```python
from build123d import *

# Parameters (mm, degrees)
F3_D     = 10
F3_DEPTH = 18


with BuildPart() as f1:
    # F0 (on Top) → F1 (revolve)
    with BuildSketch(Plane.XY):
        Polygon((0, 42.5), (0, 9), (85, 9), (85, 14), (48, 21), (18, 21), (18, 42.5), align=None)
    revolve(axis=Axis((69.263607, 0, 0), (1, 0, 0)))

    # F3
    with Locations(Plane.YZ.offset(18)):
        with Locations((0, 32.5), (-32.5, 0), (0, -32.5), (32.5, 0)):
            Hole(F3_D / 2, depth=F3_DEPTH)


solid = f1.part
```
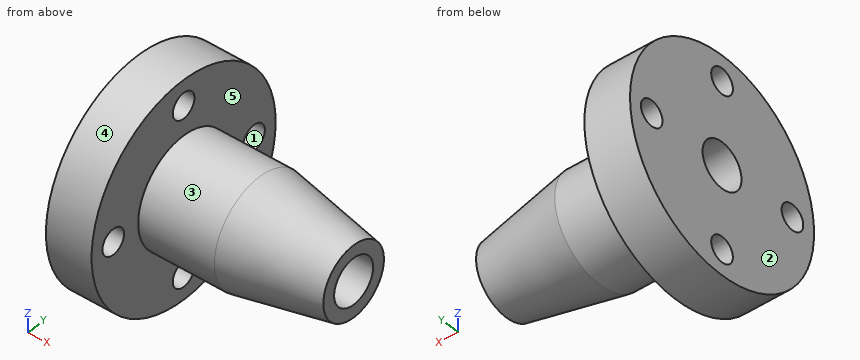
Geometry check sheet. Reference: the model listing, model coordinates, mm. Face numbers are marked on the shaded views. A direction names the side the tool comes from. Coordinates: 2 decimals unless noted, no trailing zeros. Order: outer loops, then holes, each group sorted by start corner. A loop starts at its lowest first (then second) coordinate and runs counter-clockwise, first axis right, second up. Notation, with made-up numbers: M 20.25,45 L 24.25,45 A28 cw 24.25,72 Z; hole C 6.25,2.25 d10. An arc over 180 degrees is marked long. Answer as a JSON object with one key per item and string values.
Q1. Cross-section at C-C on z = -30. Record the cut outline in (x, y).
Results are:
{"outline": "M 0,-30.1 L 18,-30.1 L 18,-4.33 L 0,-4.33 Z; M 0,4.33 L 18,4.33 L 18,30.1 L 0,30.1 Z"}
Q2. Depth check by flat-ended pin: pin 1 Ø8 at (y, z) = (0, 32.5) entering from +X; pin 2 Ø1 at (x, y) = (14, 25) entering from -Z; pin 3 Ø12 at (y, z) = (-13, -32) entering from +X; pin 4 Ø5 at (x, y) = (31.5, -11.5) entering from -Z. Enter the tip coordinate at first touch or a pass-through.
Results are:
{"pin 1": "passes through", "pin 2": "stops at z = -34.73", "pin 3": "stops at x = 18", "pin 4": "stops at z = -18.97"}
Q3. Scan lines: line 1 (Z direction, x = 10, y = 0); line 2 (X direction, y = 26, z = -26); line 3 (Z direction, x = 61.5, y = 7). Record each from-to range of solid material in increasing order.
Results are:
{"line 1": "z = -42.5 to -37.5, -27.5 to -9, 9 to 27.5, 37.5 to 42.5", "line 2": "x = 0 to 18", "line 3": "z = -17.07 to -5.66, 5.66 to 17.07"}
Q4. Cross-section at A-A on z = 0. Record the cut outline in (x, y), and give its area (4 significant figures).
Results are:
{"outline": "M 0,-42.5 L 18,-42.5 L 18,-37.5 L 0,-37.5 Z; M 0,-27.5 L 18,-27.5 L 18,-21 L 48,-21 L 85,-14 L 85,-9 L 0,-9 Z; M 0,9 L 85,9 L 85,14 L 48,21 L 18,21 L 18,27.5 L 0,27.5 Z; M 0,37.5 L 18,37.5 L 18,42.5 L 0,42.5 Z", "area": "2,195 mm²"}
Q5. Release check for a two-part mould opening along Y. For the marked faces 1, 2 and 3 record: released by +Y, released by -Y, zero draft, split by the parting line, or undercut.
Results are:
{"face 1": "undercut", "face 2": "zero draft", "face 3": "split by the parting line"}
Q6. Cross-section at D-D on x = 32. Record the cut outline in (y, z), and give its area (3 significant figures).
Results are:
{"outline": "C 0,0 d42; hole C 0,0 d18", "area": "1,130 mm²"}
Q7. Tool access check on the marked faces 4 and 5. Record the directions out of +Z, -Z, +X, -X, +Y, -Y that give a thin tool (end or side, any length) a straight path to the whole face; none if there is none.
Results are:
{"face 4": "+X, -X", "face 5": "+X"}
